The listing builds one solid part. Answer for the finished solid, in the listing's coordinates (mm). Face numbers are marked on the shaded views. A direction names the side the tool comes from. Round coordinates to 2 decimals unless told otherwise and drop trailing zeros. Write each loop counter-clockwise with the first axis right and the second up, starting at its lowest first coordinate (ties: lowest second). Pieces come first, ordered by that corner, then holes. Notation, with made-up numbers: M -1,20 L 44,20 A36 cw 44,59 Z; hole C -24.75,80 d2. An arc over 180 degrees is marked long. One line per item, written item: value. Start each with the question number.
(1) Section B-B (z = 3) is taken. Determine the outline of the cut face in (x, y), plus the area to 3 significant figures.
(2) Consider probe 1 along X at (y, z) = (0.25, 2.25); probe 2 along Y at (x, z) = (0.75, 3); probe 3 along Y at (x, z) = (12.25, 3.8). Determine where each line is inside the solid, lowest interval first.
(3) Section C-C (x = 14.25) is taken. Determine the outline of the cut face in (y, z), plus the area to 3 significant figures.
(4) For a pull along Y with two mould halves and no side action, classify the marked faces 3, 4 and 5 as released by +Y, released by -Y, zero draft, split by the parting line, or undercut.
(5) Section D-D (y = -7.1) is taken. Determine the outline of the cut face in (x, z), plus the area to 3 significant figures.
(6) Section A-A (y = 0) is taken. Determine the outline of the cut face in (x, z).
(7) For the marked faces 1 and 2, determine the directions among +Z, -Z, +X, -X, +Y, -Y from which every point of the face is accessible in a straight line to the end or side of a thin tool.
(8) Given P1, Ø0.8, axis at y = -6.5, z = 3, coming from the -X side; P2, Ø3.5, axis at y = 7.1, z = 3, coming from the +X side; P3, Ø2, axis at y = -7.1, z = 3, coming from the +X side, each flat-ended and moving along its own axis, determine where each tip first touches the part or whether it passes through.
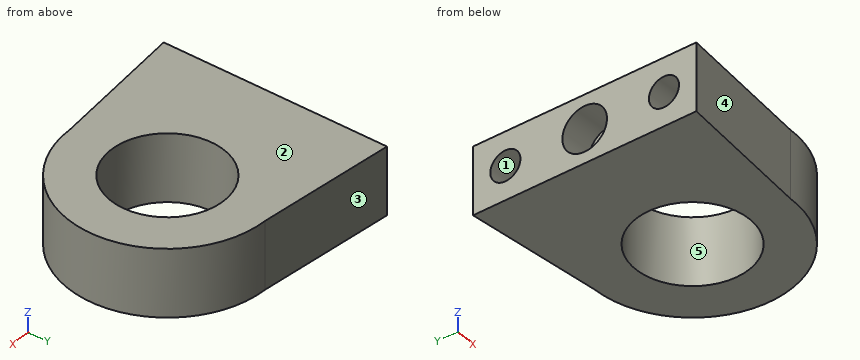
```python
from build123d import *

# Parameters (mm, degrees)
SKETCH1_R           = 5
BOSS_EXTRUDE1_DEPTH = 6
SKETCH2_R           = 1.35
SKETCH2_R_2         = 2
CUT_EXTRUDE1_DEPTH  = 3


with BuildPart() as part:
    # Sketch1 → Boss-Extrude1 (new body)
    with BuildSketch(Plane.XY):
        with BuildLine():
            Line((0, 0), (0, 10))
            Line((0, 10), (12.25, 8.75))
            ThreePointArc((12.25, 8.75), (21, 0), (12.25, -8.75))
            Line((12.25, -8.75), (0, -10))
            Line((0, -10), (0, 0))
        make_face()
        with Locations((12.25, 0)):
            Circle(SKETCH1_R, mode=Mode.SUBTRACT)
    extrude(amount=BOSS_EXTRUDE1_DEPTH)

    # Sketch2 → Cut-Extrude1 (cut)
    with BuildSketch(Plane.ZY):
        with Locations((3, 7.1)):
            Circle(SKETCH2_R)
        with Locations((3, -7.1)):
            Circle(SKETCH2_R)
        with Locations((3, 0)):
            Circle(SKETCH2_R_2)
    extrude(amount=-CUT_EXTRUDE1_DEPTH, mode=Mode.SUBTRACT)


solid = part.part
```
Recorded:
1. outline: M 0,-10 L 12.25,-8.75 A8.75 ccw 12.25,8.75 L 0,10 L 0,8.45 L 3,8.45 L 3,5.75 L 0,5.75 L 0,2 L 3,2 L 3,-2 L 0,-2 L 0,-5.75 L 3,-5.75 L 3,-8.45 L 0,-8.45 Z; hole C 12.25,0 d10
1. area: 243 mm2
2. probe 1: x = 3 to 7.26, 17.24 to 21
2. probe 2: y = -9.92 to -8.45, -5.75 to -2, 2 to 5.75, 8.45 to 9.92
2. probe 3: y = -8.75 to -5, 5 to 8.75
3. outline: M -8.52,0 L -4.58,0 L -4.58,6 L -8.52,6 Z; M 4.58,0 L 8.52,0 L 8.52,6 L 4.58,6 Z
3. area: 47.2 mm2
4. face 3: released by +Y
4. face 4: released by -Y
4. face 5: undercut
5. outline: M 0,0 L 17.36,0 L 17.36,6 L 0,6 L 0,4.35 L 3,4.35 L 3,1.65 L 0,1.65 Z
5. area: 96.1 mm2
6. outline: M 0,0 L 7.25,0 L 7.25,6 L 0,6 L 0,5 L 3,5 L 3,1 L 0,1 Z; M 17.25,0 L 21,0 L 21,6 L 17.25,6 Z
7. face 1: -X
7. face 2: +Z, +X, -X, +Y, -Y
8. P1: stops at x = 3
8. P2: stops at x = 19.17
8. P3: stops at x = 18.52
